from build123d import *

# Parameters (mm, degrees)
F1_R     = 6.75
F2_DEPTH = 15
F3_R     = 9
F4_DEPTH = 45
F5_W     = 35
F5_H     = 35
F5_R     = 9
F6_DEPTH = 6
F7_R     = 1.4
F8_DEPTH = 15


with BuildPart() as f2:
    # F1 (on offset) → F2 (new body)
    with BuildSketch(Plane.XY.offset(40)):
        Circle(F1_R)
    extrude(amount=-F2_DEPTH)

    # F3 (on offset) → F4 (join)
    with BuildSketch(Plane.XY.offset(40)):
        Circle(F3_R)
    extrude(amount=F4_DEPTH)

    # F5 (on face) → F6 (join)
    with BuildSketch(Plane.XY.offset(85)):
        with Locations((0, -3.5)):
            Rectangle(F5_W, F5_H)
        Circle(F5_R, mode=Mode.SUBTRACT)
    extrude(amount=-F6_DEPTH)

    # F7 (on face) → F8 (cut)
    with BuildSketch(Plane(origin=(0, 14, 0), x_dir=(-1, 0, 0), z_dir=(0, 1, 0))):
        with Locations((-10, 82)):
            Circle(F7_R)
        with Locations((10, 82)):
            Circle(F7_R)
    extrude(amount=-F8_DEPTH, mode=Mode.SUBTRACT)


solid = f2.part
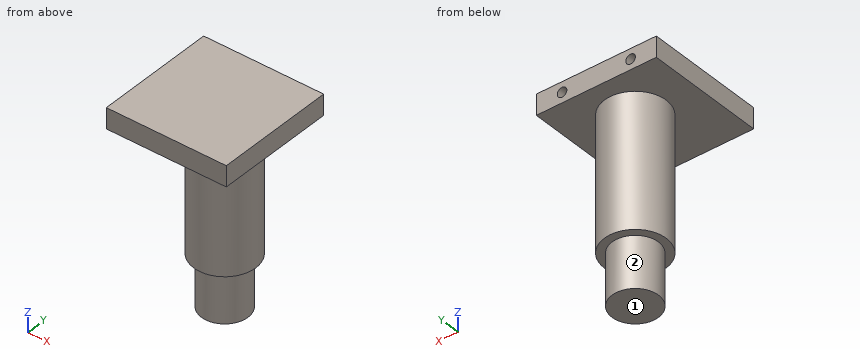
The model under review builds one solid part; all positions refer to its coordinate system, in mm. Face numbers are marked on the shaded views. A direction names the side the tool comes from. Give positions to 0.01 mm unless a question says otherwise; leave off trailing zeros. Loops run counter-clockwise (first coordinate to the right, second up) from the corner with the lowest first, then second, coordinate; pieces in that order, holes last. Notation, with made-up numbers: (39, 0) -> (65, 0) arc R36 cw to (65, 38) -> close; hole circle Ø10 at (-9, -27.5). An arc over 180 degrees is marked (long way). Answer as a JSON object with one key per item and string values. Group by question number.
Q1. Take a section at D-D (y = -4). Write out the cut boundary in (x, z).
Q2. Take a section at B-B (x = 10). Write out the cut boundary in (y, z).
Q3. Tool access review of the marked faces 1 and 2: name each direction out of +Z, -Z, +X, -X, +Y, -Y from which nothing blocks a thin tool from reaching the whole face with its end or side.
Q4. Insertion check: pin 1 (1.5 mm diameter, centred on x = -10, z = 47, fed in from -Y); pin 2 (0.8 mm diameter, centred on x = 10.5, z = 81.5, fed in from +Y); pin 3 (2 mm diameter, centred on y = -1, z = 55, fed in from -X); pin 4 (6 mm diameter, centred on x = 4, z = 47, fed in from -Y). Each pin has a flat end and moves straight along its axis. Give the tip position at first contact, or say it passes through.
Q5. Take a section at C-C (y = 0). Write out the cut boundary in (x, z).
Q6. Wall thickness on line 1 along X through (y, z) = (5, 82); line 2 along Z through (x, y) = (10, 5.25); line 3 along Z through (x, y) = (-13.5, 2): over which ranges is each line inside the solid? List them lowest first.
Q7. Take a section at A-A (z = 82). Write out the cut boundary in (x, y), plus the area to 3 significant figures.
Answer below:
{
 "1": {"outline": "(-17.5, 79) -> (-8.06, 79) -> (-8.06, 40) -> (-5.44, 40) -> (-5.44, 25) -> (5.44, 25) -> (5.44, 40) -> (8.06, 40) -> (8.06, 79) -> (17.5, 79) -> (17.5, 85) -> (-17.5, 85) -> close"},
 "2": {"outline": "(-21, 79) -> (14, 79) -> (14, 80.6) -> (-1, 80.6) -> (-1, 83.4) -> (14, 83.4) -> (14, 85) -> (-21, 85) -> close"},
 "3": {"face 1": "-Z, +X, -X, +Y, -Y", "face 2": "-Z"},
 "4": {"pin 1": "passes through", "pin 2": "stops at y = -1", "pin 3": "stops at x = -9", "pin 4": "stops at y = -8.94"},
 "5": {"outline": "(-17.5, 79) -> (-9, 79) -> (-9, 40) -> (-6.75, 40) -> (-6.75, 25) -> (6.75, 25) -> (6.75, 40) -> (9, 40) -> (9, 79) -> (17.5, 79) -> (17.5, 85) -> (-17.5, 85) -> close; hole circle Ø2.8 at (-10, 82); hole circle Ø2.8 at (10, 82)"},
 "6": {"line 1": "x = -17.5 to -11.4, -8.6 to 8.6, 11.4 to 17.5", "line 2": "z = 79 to 80.6, 83.4 to 85", "line 3": "z = 79 to 85"},
 "7": {"outline": "(-17.5, -21) -> (17.5, -21) -> (17.5, 14) -> (11.4, 14) -> (11.4, -1) -> (8.6, -1) -> (8.6, 14) -> (-8.6, 14) -> (-8.6, -1) -> (-11.4, -1) -> (-11.4, 14) -> (-17.5, 14) -> close", "area": "1,140 mm2"}
}
